Geometry: final body of the model. Coordinates: model frame, mm. Face numbers are marked on the shaded views. A direction names the side the tool comes from. Give positions to 0.01 mm unless a question says otherwise; leave off trailing zeros. Write each loop counter-clockwise with the first axis right and the second up, starting at its lowest first coordinate (ties: lowest second). Pieces come first, ordered by that corner, then holes. Notation, with made-up numbers: M -11.75,8 L -4.75,8 A26 ccw -4.75,27 Z; hole C 28.5,58 d1. An arc over 180 degrees is marked long. Use a Markdown table: item, result. Add a question column.
1) Pin query (flat end, axial travel): pin 1 (2 mm diameter, centred on x = -4.5, z = 2, fed in from -Y); pin 2 (1 mm diameter, centred on x = 1, y = 6, fed in from +Z). Return the tip coordinate at first contact, or that it passes through.
2) Line query: line 1 (Z direction, x = 1, y = 5.75); line 2 (Z direction, x = 3, y = 4.5); line 3 (X direction, y = -5.75, z = 1.55). Output: solid intervals per line, ascending.
3) Section C-C on z = 1.4. Return the cut outline in (x, y), then the cut area to 3 significant figures.
4) Set-up query: the marked faces 1 and 2. Return all of +Z, -Z, +X, -X, +Y, -Y with unobstructed straight access to the full face (end or side cutting, diameter ignored); none if empty.
5) Section A-A on y = 0. Return the cut outline in (x, z).
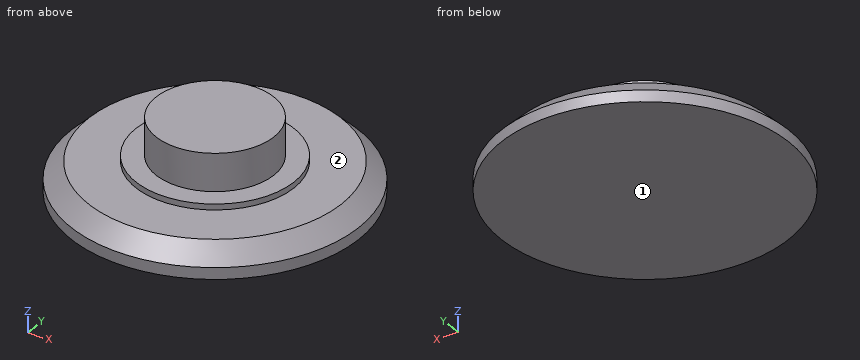
```python
from build123d import *

# Parameters (mm, degrees)
F0_R     = 10
F0_R_2   = 5.5
F0_R_3   = 4.1
F1_DEPTH = 2
F2_DEPTH = 5
F3_SIZE  = 1.2
F4_DEPTH = 2.4


with BuildPart() as f1:
    # F0 (on Top) → F1 (new body)
    with BuildSketch(Plane.XY):
        Circle(F0_R)
        Circle(F0_R_2, mode=Mode.SUBTRACT)
        Circle(F0_R_3)
        Circle(F0_R_2)
        Circle(F0_R_3, mode=Mode.SUBTRACT)
    extrude(amount=F1_DEPTH)

    # F0 (on Top) → F2 (join)
    with BuildSketch(Plane.XY):
        Circle(F0_R_3)
    extrude(amount=F2_DEPTH)

    # F3
    f3_edges = [f1.edges().sort_by_distance(p)[0] for p in [
        (-10, 0, 2),
    ]]
    chamfer(f3_edges, length=F3_SIZE)

    # F0 (on Top) → F4 (join)
    with BuildSketch(Plane.XY):
        Circle(F0_R_2)
        Circle(F0_R_3, mode=Mode.SUBTRACT)
    extrude(amount=F4_DEPTH)


solid = f1.part
```
Found:
| question | item | result |
|---|---|---|
| 1 | pin 1 | y = -8.81 |
| 1 | pin 2 | z = 2 |
| 2 | line 1 | 0 to 2 |
| 2 | line 2 | 0 to 2.4 |
| 2 | line 3 | -7.25 to 7.25 |
| 3 | outline | C 0,0 d18.8 |
| 3 | area | 278 mm² |
| 4 | face 1 | -Z, +X, -X, +Y, -Y |
| 4 | face 2 | +Z |
| 5 | outline | M -10,0 L 10,0 L 10,0.8 L 8.8,2 L 5.5,2 L 5.5,2.4 L 4.1,2.4 L 4.1,5 L -4.1,5 L -4.1,2.4 L -5.5,2.4 L -5.5,2 L -8.8,2 L -10,0.8 Z |
